```python
from build123d import *

# Parameters (mm, degrees)
F0_R     = 65.066172
F1_DEPTH = 38.1
F2_R     = 38.1
F2_R_2   = 9.525
F3_DEPTH = 158.496
F4_R     = 6.537094
F5_DEPTH = 155.702
F6_W     = 100.18133
F6_H     = 22.402564
F7_DEPTH = 38.101
F8_W     = 11.216447
F8_H     = 17.543803
F9_DEPTH = 84.131507


with BuildPart() as f1:
    # F0 (on Front) → F1 (new body)
    with BuildSketch(Plane.XZ):
        Circle(F0_R)
    extrude(amount=F1_DEPTH)

    # F2 (on face) → F3 (join)
    with BuildSketch(Plane.XZ.offset(38.1)):
        Circle(F2_R)
        with Locations((15.875, 0)):
            Circle(F2_R_2, mode=Mode.SUBTRACT)
    extrude(amount=F3_DEPTH)

    # F4 (on face) → F5 (join)
    with BuildSketch(Plane.XZ.offset(38.1)):
        with Locations((-37.386458, 33.612467)):
            Circle(F4_R)
    extrude(amount=F5_DEPTH)

    # F6 (on face) → F7 (cut, through all)
    with BuildSketch(Plane.XZ.offset(38.1)):
        with Locations((85.523775, 30.265617)):
            Rectangle(F6_W, F6_H)
    extrude(amount=-F7_DEPTH, mode=Mode.SUBTRACT)

    # F8 (on face) → F9 (cut, through all)
    with BuildSketch(Plane.XY.offset(19.064335)):
        with Locations((52.434615, -17.852365)):
            Rectangle(F8_W, F8_H)
    extrude(amount=-F9_DEPTH, mode=Mode.SUBTRACT)


solid = f1.part
```
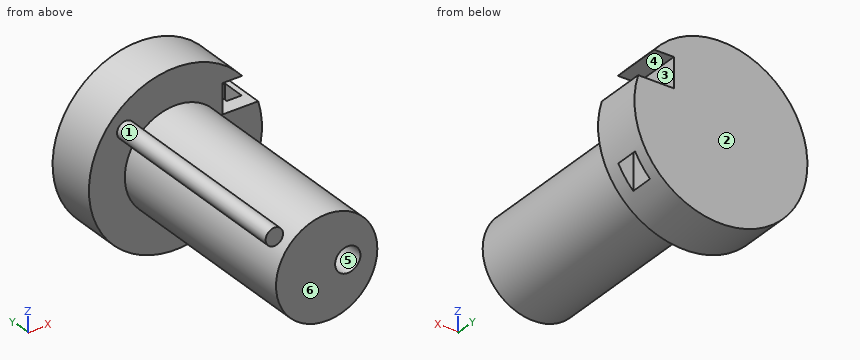
Check sheet for the modelled part. Datum: model origin and axes. Units: mm. Face numbers are marked on the shaded views. A direction names the side the tool comes from. Round coordinates to 2 decimals unless told otherwise and drop trailing zeros. Order: outer loops, then holes, each group sorted by start corner. A loop starts at its lowest first (then second) coordinate and runs counter-clockwise, first axis right, second up.
1) Section check B-B (x = 1). Record the boundary of the cut face in (y, z), and give its area (3 significant figures).
2) Section check D-D (z = 48). Record the boundary of the cut face in (x, y).
3) Section check C-C (y = -126.5). Record the boundary of the cut face in (x, z) (3 decimals).
4) Section check A-A (z = 0). Record the boundary of the cut face in (x, y).
5) Go/stop test with flat-tipped pins: pin 1 Ø10.5 at (x, z) = (-35.5, 33.5) entering from -Y; pin 2 Ø2 at (x, y) = (-20.5, -41.5) entering from -Z; pin 3 Ø8 at (x, y) = (53, -19.5) entering from +Z. Record where each tip stops, or that it passes through.
6) Tool access check on the marked faces 4, 5 and 6. Record the directions out of +Z, -Z, +X, -X, +Y, -Y that give a thin tool (end or side, any length) a straight path to the whole face; none if there is none.
7) Scan lines: line 1 (Y direction, x = -33.5, z = 32); line 2 (Z direction, x = 14, y = -135.5); line 3 (Y direction, x = -8, z = -53.5). Record each from-to range of solid material in increasing order.
8) Mould release check, pull along X, two halves, no side actions. Record for the marked faces 1, 2 and 3: +X half, -X half, draft (parallel to the pull), parting line (faces both ways), or undercut.
Result:
1. outline: (-196.6, -38.09) - (-38.1, -38.09) - (-38.1, -65.06) - (0, -65.06) - (0, 65.06) - (-38.1, 65.06) - (-38.1, 38.09) - (-196.6, 38.09) - close
1. area: 17,000 mm2
2. outline: (-43.93, -38.1) - (43.93, -38.1) - (43.93, 0) - (-43.93, 0) - close
3. outline: circle Ø13.074 at (-37.386, 33.612); circle Ø76.2 at (0, 0); hole circle Ø19.05 at (15.875, 0)
4. outline: (-65.07, -38.1) - (-38.1, -38.1) - (-38.1, -196.6) - (6.35, -196.6) - (6.35, -38.1) - (25.4, -38.1) - (25.4, -196.6) - (38.1, -196.6) - (38.1, -38.1) - (65.07, -38.1) - (65.07, 0) - (-65.07, 0) - close; hole (46.83, -26.62) - (58.04, -26.62) - (58.04, -9.08) - (46.83, -9.08) - close
5. pin 1: stops at y = -193.8
5. pin 2: stops at z = -32.73
5. pin 3: stops at z = 42.81
6. face 4: +X, +Y, -Y
6. face 5: -Y
6. face 6: +Z, -Z, +X, -X, -Y
7. line 1: y = -193.8 to 0
7. line 2: z = -35.43 to -9.34, 9.34 to 35.43
7. line 3: y = -38.1 to 0
8. face 1: undercut
8. face 2: draft
8. face 3: +X half
